from build123d import *

# Parameters (mm, degrees)
SKETCH_2_R          = 11
EXTRUDE_1_DEPTH     = 16
EXTRUDE_2_DEPTH     = 14
SKETCH_5_R          = 10.75
EXTRUDE_3_DEPTH     = 120
EXTRUDE_4_DEPTH     = 14
SKETCH_7_R          = 8
CUT_EXTRUDE_1_DEPTH = 3
SKETCH_8_R          = 4
CUT_EXTRUDE_2_DEPTH = 100
SKETCH_9_R          = 5
CUT_EXTRUDE_3_DEPTH = 15
SKETCH_10_R         = 11
EXTRUDE_5_DEPTH     = 22
CHAMFER_1_SIZE      = 6
CUT_EXTRUDE_START   = -22
CUT_EXTRUDE_4_DEPTH = 22
SKETCH_12_R         = 3.5
CUT_EXTRUDE_5_DEPTH = 188.704555105


with BuildPart() as part:
    # ｽｹｯﾁ2 → ﾎﾞｽ - 押し出し1 (new body)
    with BuildSketch(Plane(origin=(0, 0, 0), x_dir=(0, 0, -1), z_dir=(1, 0, 0))):
        Circle(SKETCH_2_R)
    extrude(amount=EXTRUDE_1_DEPTH)

    # ｽｹｯﾁ4 → ﾎﾞｽ - 押し出し2 (add)
    with BuildSketch(Plane(origin=(16, 0, 0), x_dir=(0, 0, -1), z_dir=(1, 0, 0))):
        with BuildLine():
            Line((13, -5.196152423), (13, 5.196152423))
            Line((13, 5.196152423), (9.695359715, 5.196152423))
            ThreePointArc((9.695359715, 5.196152423), (10.668855535, 2.678716403), (11, 0))
            ThreePointArc((11, 0), (10.668855535, -2.678716403), (9.695359715, -5.196152423))
            Line((9.695359715, -5.196152423), (13, -5.196152423))
        make_face()
        with BuildLine():
            Line((9.695359715, 5.196152423), (-9.695359715, 5.196152423))
            ThreePointArc((-9.695359715, 5.196152423), (-11, 0), (-9.695359715, -5.196152423))
            Line((-9.695359715, -5.196152423), (9.695359715, -5.196152423))
            ThreePointArc((9.695359715, -5.196152423), (10.668855535, -2.678716403), (11, 0))
            ThreePointArc((11, 0), (10.668855535, 2.678716403), (9.695359715, 5.196152423))
        make_face()
        with BuildLine():
            Line((-9.695359715, 5.196152423), (-13, 5.196152423))
            Line((-13, 5.196152423), (-13, -5.196152423))
            Line((-13, -5.196152423), (-9.695359715, -5.196152423))
            ThreePointArc((-9.695359715, -5.196152423), (-11, 0), (-9.695359715, 5.196152423))
        make_face()
        with BuildLine():
            ThreePointArc((13, 5.196152423), (0, 14), (-13, 5.196152423))
            Line((-13, 5.196152423), (-9.695359715, 5.196152423))
            ThreePointArc((-9.695359715, 5.196152423), (0, 11), (9.695359715, 5.196152423))
            Line((9.695359715, 5.196152423), (13, 5.196152423))
        make_face()
        with BuildLine():
            ThreePointArc((9.695359715, 5.196152423), (0, 11), (-9.695359715, 5.196152423))
            Line((-9.695359715, 5.196152423), (9.695359715, 5.196152423))
        make_face()
        with BuildLine():
            Line((9.695359715, -5.196152423), (-9.695359715, -5.196152423))
            ThreePointArc((-9.695359715, -5.196152423), (0, -11), (9.695359715, -5.196152423))
        make_face()
        with BuildLine():
            Line((-9.695359715, -5.196152423), (-13, -5.196152423))
            ThreePointArc((-13, -5.196152423), (0, -14), (13, -5.196152423))
            Line((13, -5.196152423), (9.695359715, -5.196152423))
            ThreePointArc((9.695359715, -5.196152423), (0, -11), (-9.695359715, -5.196152423))
        make_face()
    extrude(amount=EXTRUDE_2_DEPTH)

    # ｽｹｯﾁ5 → ﾎﾞｽ - 押し出し3 (add)
    with BuildSketch(Plane(origin=(30, 0, 0), x_dir=(0, 0, -1), z_dir=(1, 0, 0))):
        Circle(SKETCH_5_R)
    extrude(amount=EXTRUDE_3_DEPTH)

    # ｽｹｯﾁ6 → ﾎﾞｽ - 押し出し4 (add)
    with BuildSketch(Plane(origin=(150, 0, 0), x_dir=(0, 0, -1), z_dir=(1, 0, 0))):
        with BuildLine():
            ThreePointArc((9.410765112, 5.196152423), (0, 10.75), (-9.410765112, 5.196152423))
            Line((-9.410765112, 5.196152423), (9.410765112, 5.196152423))
        make_face()
        with BuildLine():
            ThreePointArc((13, 5.196152423), (0, 14), (-13, 5.196152423))
            Line((-13, 5.196152423), (-9.410765112, 5.196152423))
            ThreePointArc((-9.410765112, 5.196152423), (0, 10.75), (9.410765112, 5.196152423))
            Line((9.410765112, 5.196152423), (13, 5.196152423))
        make_face()
        with BuildLine():
            ThreePointArc((-9.410765112, 5.196152423), (-10.75, 0), (-9.410765112, -5.196152423))
            Line((-9.410765112, -5.196152423), (9.410765112, -5.196152423))
            ThreePointArc((9.410765112, -5.196152423), (10.409808475, -2.682981088), (10.75, 0))
            ThreePointArc((10.75, 0), (10.409808475, 2.682981088), (9.410765112, 5.196152423))
            Line((9.410765112, 5.196152423), (-9.410765112, 5.196152423))
        make_face()
        with BuildLine():
            Line((9.410765112, -5.196152423), (13, -5.196152423))
            Line((13, -5.196152423), (13, 5.196152423))
            Line((13, 5.196152423), (9.410765112, 5.196152423))
            ThreePointArc((9.410765112, 5.196152423), (10.409808475, 2.682981088), (10.75, 0))
            ThreePointArc((10.75, 0), (10.409808475, -2.682981088), (9.410765112, -5.196152423))
        make_face()
        with BuildLine():
            Line((-13, 5.196152423), (-13, -5.196152423))
            Line((-13, -5.196152423), (-9.410765112, -5.196152423))
            ThreePointArc((-9.410765112, -5.196152423), (-10.75, 0), (-9.410765112, 5.196152423))
            Line((-9.410765112, 5.196152423), (-13, 5.196152423))
        make_face()
        with BuildLine():
            Line((9.410765112, -5.196152423), (-9.410765112, -5.196152423))
            ThreePointArc((-9.410765112, -5.196152423), (0, -10.75), (9.410765112, -5.196152423))
        make_face()
        with BuildLine():
            Line((-9.410765112, -5.196152423), (-13, -5.196152423))
            ThreePointArc((-13, -5.196152423), (0, -14), (13, -5.196152423))
            Line((13, -5.196152423), (9.410765112, -5.196152423))
            ThreePointArc((9.410765112, -5.196152423), (0, -10.75), (-9.410765112, -5.196152423))
        make_face()
    extrude(amount=EXTRUDE_4_DEPTH)

    # ｽｹｯﾁ7 → ｶｯﾄ - 押し出し1 (cut)
    with BuildSketch(Plane.ZY):
        Circle(SKETCH_7_R)
    extrude(amount=-CUT_EXTRUDE_1_DEPTH, mode=Mode.SUBTRACT)

    # ｽｹｯﾁ8 → ｶｯﾄ - 押し出し2 (cut)
    with BuildSketch(Plane.ZY.offset(-3)):
        Circle(SKETCH_8_R)
    extrude(amount=-CUT_EXTRUDE_2_DEPTH, mode=Mode.SUBTRACT)

    # ｽｹｯﾁ9 → ｶｯﾄ - 押し出し3 (cut)
    with BuildSketch(Plane(origin=(0, 20, 0), x_dir=(1, 0, 0), z_dir=(0, 1, 0))):
        with Locations(Location((23, 0, 0), (0, 0, 270))):
            Circle(SKETCH_9_R)
        with Locations(Location((157, 0, 0), (0, 0, 270))):
            Circle(SKETCH_9_R)
    extrude(amount=-CUT_EXTRUDE_3_DEPTH, mode=Mode.SUBTRACT)

    # ｽｹｯﾁ10 → ﾎﾞｽ - 押し出し5 (add)
    with BuildSketch(Plane(origin=(164, 0, 0), x_dir=(0, 0, -1), z_dir=(1, 0, 0))):
        Circle(SKETCH_10_R)
    extrude(amount=EXTRUDE_5_DEPTH)

    # 面取り1
    chamfer_1_edges = [part.edges().sort_by_distance(p)[0] for p in [
        (186, 0, 11),
    ]]
    chamfer(chamfer_1_edges, length=CHAMFER_1_SIZE)

    # ｽｹｯﾁ11 → ｶｯﾄ - 押し出し4 (cut)
    with BuildSketch(Plane(origin=(186, 0, 0), x_dir=(0, 0, -1), z_dir=(1, 0, 0)).offset(CUT_EXTRUDE_START)):
        with BuildLine():
            ThreePointArc((-8, 7.549834435), (-11, 0), (-8, -7.549834435))
            Line((-8, -7.549834435), (-8, 7.549834435))
        make_face()
        with BuildLine():
            Line((8, 7.549834435), (8, -7.549834435))
            ThreePointArc((8, -7.549834435), (10.22252415, -4.062019202), (11, 0))
            ThreePointArc((11, 0), (10.22252415, 4.062019202), (8, 7.549834435))
        make_face()
    extrude(amount=CUT_EXTRUDE_4_DEPTH, mode=Mode.SUBTRACT)

    # ｽｹｯﾁ12 → ｶｯﾄ - 押し出し5 (cut, through all)
    with BuildSketch(Plane.XY.offset(8)):
        with Locations((176, 0)):
            Circle(SKETCH_12_R)
    extrude(amount=-CUT_EXTRUDE_5_DEPTH, mode=Mode.SUBTRACT)


solid = part.part
Here's how the part is built. I have some questions about the finished solid (model axes, mm). A direction names the side the tool comes from. Give positions to 0.01 mm unless a question says otherwise; leave off trailing zeros. Order: outer loops, then holes, each group sorted by start corner. A loop starts at its lowest first (then second) coordinate and runs counter-clockwise, first axis right, second up. Notation, with made-up numbers: (-18.5, 88) -> (5.5, 88) arc R10 ccw to (5.5, 99) -> close; hole circle Ø10 at (51, -0.5). An arc over 180 degrees is marked (long way). One line per item, written item: value. Start each with the question number.
1. I need wall thicknesses on probe 1 along Y at (x, z) = (44.5, -0.25); probe 2 along X at (y, z) = (7.5, -10.5); probe 3 along X at (y, z) = (9.25, 0). Which ranges of each line are inside material? Lowest first, please. Write a range as from..to.
2. Imagine slicing it at C-C, the plane x = 23. List the corners of the cut face in (y, z) for me.
3. Imagine slicing it at B-B, the plane x = 176. List the corners of the cut face in (y, z) for me, plus the area to 3 significant figures.
4. Imagine slicing it at D-D, the plane x = 155. List the corners of the cut face in (y, z) for me.
5. For faces 4 (the face through (172, -11, 0)), 5 (the face through (23, 5, 0)), 6 (the face through (171, 0, -8)), 7 (the face through (171, 0, 8)), 8 (the face through (7.89, -10.74, 2.38)), which set-ups out of +Z, -Z, +X, -X, +Y, -Y let a thin tool reach every point of the face, with its end or its side?
6. We'd pull the mould along Y, two halves only. Please class faces 1 (the face through (103, 0, 0)), 2 (the face through (157, 0, 13)), 3 (the face through (18.24, 13.45, -3.89)): released by +Y, released by -Y, zero draft, split by the parting line, or undercut.
7. Will these pins go through, and if not, where does the flat tip stop? pin 1 Ø6 at (x, y) = (109, 3) entering from +Z; pin 2 Ø10 at (x, z) = (90.5, -4.5) entering from -Y; pin 3 Ø8 at (y, z) = (1, 3.5) entering from -X.
Values follow:
1. probe 1: y = -10.75..-3.99, 3.99..10.75
1. probe 2: x = 16..30, 150..164
1. probe 3: x = 0..18, 28..152, 162..181.75
2. outline: (-5.2, -13) -> (5.2, -13) arc R14 ccw to (13.08, -5) -> (5, -5) -> (5, 5) -> (13.08, 5) arc R14 ccw to (5.2, 13) -> (-5.2, 13) arc R14 ccw to start; hole circle Ø8 at (0, 0)
3. outline: (-7.55, -8) -> (-3.5, -8) -> (-3.5, 8) -> (-7.55, 8) arc R11 ccw to start; (3.5, -8) -> (7.55, -8) arc R11 ccw to (7.55, 8) -> (3.5, 8) -> close
3. area: 206 mm2
4. outline: (-5.2, -13) -> (5.2, -13) arc R14 ccw to (13.23, -4.58) -> (5, -4.58) -> (5, 4.58) -> (13.23, 4.58) arc R14 ccw to (5.2, 13) -> (-5.2, 13) arc R14 ccw to start
5. face 4: +X, -Y
5. face 5: +Y
5. face 6: -Z, +X, +Y, -Y
5. face 7: +Z, +X, +Y, -Y
5. face 8: -X
6. face 1: undercut
6. face 2: zero draft
6. face 3: released by +Y
7. pin 1: stops at z = 10.75
7. pin 2: stops at y = -10.75
7. pin 3: stops at x = 3
